The listing builds one solid part. Answer for the finished solid, in the listing's coordinates (mm). Give positions to 0.01 mm unless a question says otherwise; leave off trailing zeros. Write each loop counter-clockwise with the first axis right and the second up, starting at its lowest first coordinate (ties: lowest second). Pieces come first, ordered by that corner, then holes. Notation, with made-up numbers: (9.25, 25.25) - (42.25, 25.25) arc R17 cw to (42.25, 51.25) - close; hole circle Ø5 at (71.25, 84). An arc over 180 degrees is marked (long way). Return JSON: item names as keys, results as strings.
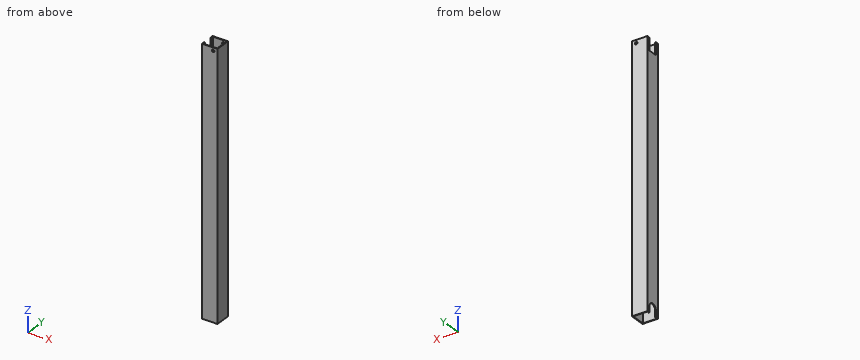
Autodesk Inventor part; units mm, degrees
ref_plane "Work Plane3" through (15.875, 0, 0) normal (1, 0, 0) x (0, 1, 0)
ref_plane "XZ Plane" through (0, 0, 0) normal (0, 1, 0) x (-1, 0, 0)
ref_plane "XY Plane" through (0, 0, 0) normal (0, 0, 1) x (1, 0, 0)
sketch "Sketch1" plane through (0, 0, 0) normal (0, 0, 1) x (1, 0, 0)
  line L0 (0, 0) -> (31.75, 0)
  line L1 (31.75, 0) -> (31.75, 31.75)
  line L2 (31.75, 31.75) -> (0, 31.75)
  line L3 (0, 31.75) -> (0, 0)
  line L4 (1.5875, 30.1625) -> (30.1625, 30.1625)
  line L5 (30.1625, 30.1625) -> (30.1625, 1.5875)
  line L6 (30.1625, 1.5875) -> (1.5875, 1.5875)
  line L7 (1.5875, 1.5875) -> (1.5875, 30.1625)
  dimension "d0" = 31.75
  dimension "d1" = 31.75
  dimension "d2" = 1.5875
extrude "Extrusion1" add sketch "Sketch1" along normal blind 533.4
sketch "Sketch5" plane through (31.75, 0, 0) normal (1, 0, 0) x (0, 0, -1)
  line L0 (0, 15.875) -> (-12.7, 15.875) construction
  line L1 (0, 6.35) -> (-12.7, 6.35)
  line L2 (-12.7, 25.4) -> (0, 25.4)
  arc A0 (0, 6.35) -> (0, 25.4) centre (0, 15.875) ccw
  arc A1 (-12.7, 25.4) -> (-12.7, 6.35) centre (-12.7, 15.875) ccw
  line L3 (0, 0) -> (0, 31.75)
  line L4 (0, 31.75) -> (-533.4, 31.75)
  point P0 (-6.35, 15.875)
  dimension "d26" = 0
  dimension "d27" = 19.05
  dimension "d28" = 15.875
  dimension "d29" = 12.7
extrude "Extrusion4" cut sketch "Sketch5" against normal blind 25.4
ref_plane "Work Plane3" through (15.875, 0, 0) normal (1, 0, 0) x (0, 1, 0)
mirror "Mirror1" about plane through (15.875, 0, 0) normal (1, 0, 0) of "Extrusion4"
sketch "Sketch6" plane through (31.75, 0, 533.4) normal (1, 0, 0) x (0, 0, -1)
  line L0 (533.4, 25.4) -> (520.7, 25.4)
  line L1 (533.4, 25.4) -> (520.7, 25.4)
  arc A0 (520.7, 25.4) -> (520.7, 6.35) centre (520.7, 15.875) ccw
  arc A1 (520.7, 25.4) -> (520.7, 6.35) centre (520.7, 15.875) ccw
  line L2 (533.4, 6.35) -> (520.7, 6.35)
  line L3 (520.7, 6.35) -> (533.4, 6.35)
  line L4 (533.4, 25.4) -> (533.4, 31.75)
  line L5 (533.4, 25.4) -> (533.4, 6.35)
  point P0 (533.4, 0)
extrude "Extrusion5" add sketch "Sketch6" against normal blind 1.5875
sketch "Sketch8" plane through (0, 31.75, 0) normal (0, 1, 0) x (1, 0, 0)
  line L0 (31.75, 0) -> (31.75, -533.4)
  line L1 (31.75, -533.4) -> (0, -533.4)
  point P0 (0, 0)
  point P1 (23.0188, -527.05)
  dimension "d44" = 8.7312
  dimension "d45" = 6.35
hole "Hole3" at (23.0187, 31.75, 527.05) direction (0, -1, 0) diameter 5.1562 depth 76.2 tip angle 118
sketch "Sketch9" plane through (0, 0, 533.4) normal (-1, 0, 0) x (0, 0, 1)
  line L0 (0, 1.5875) -> (0, 30.1625)
  line L1 (0, 25.4) -> (-25.4, 25.4)
  line L2 (-25.4, 25.4) -> (-25.4, 6.35)
  line L3 (-25.4, 6.35) -> (0, 6.35)
  line L4 (0, 6.35) -> (0, 25.4)
  line L5 (-533.4, 0) -> (0, 0)
  line L6 (-533.4, 31.75) -> (0, 31.75)
  dimension "d53" = 25.4
  dimension "d54" = 6.35
  dimension "d55" = 6.35
extrude "Extrusion6" cut sketch "Sketch9" against normal blind 5.842
equation "\"d55\" = d54"
properties part number "TelescopeMiddleNoSlot" material "Aluminum 6061"
Item 1: Consider L1, parallel to Y at x = 16.5, z = 492.5; L2, parallel to X at y = 0.75, z = 527.05. Determine where each line is inside the solid, lowest interval first.
Answer below:
{"L1": "y = 0 to 1.59, 30.16 to 31.75", "L2": "x = 0 to 20.44, 25.6 to 31.75"}
Item 2: Flat-ended cylindrical pins translate along their axes: P1, Ø3, axis at x = 23.02, z = 527.05, coming from the +Y side; P2, Ø0.5, axis at x = 1, y = 12, coming from the +Z side. Find the tip coordinate at first contact, or state that the pin passes through.
Answer below:
{"P1": "passes through", "P2": "stops at z = 508"}
Item 3: A cutting plane is placed at A-A on z = 287. Determine the outline of the cut face in (x, y).
Answer below:
{"outline": "(0, 0) - (31.75, 0) - (31.75, 31.75) - (0, 31.75) - close; hole (1.59, 1.59) - (30.16, 1.59) - (30.16, 30.16) - (1.59, 30.16) - close"}
Item 4: A cutting plane is placed at B-B on x = 12. Determine the outline of the cut face in (y, z).
Answer below:
{"outline": "(0, 0) - (1.59, 0) - (1.59, 533.4) - (0, 533.4) - close; (30.16, 0) - (31.75, 0) - (31.75, 533.4) - (30.16, 533.4) - close"}
